from build123d import *

# Parameters (mm, degrees)
EXTRUDE_THIN1_DEPTH = 101.6
CUT_EXTRUDE1_DEPTH  = 49.784
LPATTERN1_COUNT     = 4
LPATTERN1_PITCH     = 20.32


with BuildPart() as part:
    # Sketch1 → Extrude-Thin1 (new body)
    with BuildSketch(Plane.XY):
        with BuildLine():
            Line((0, 0), (9.525, 0))
            ThreePointArc((9.525, 0), (11.77006403, 0.92993597), (12.7, 3.175))
            Line((12.7, 3.175), (12.7, 7.984742102))
            ThreePointArc((12.7, 7.984742102), (13.62993597, 10.229806132), (15.875, 11.159742102))
            Line((15.875, 11.159742102), (85.725, 11.159742102))
            ThreePointArc((85.725, 11.159742102), (87.97006403, 10.229806132), (88.9, 7.984742102))
            Line((88.9, 7.984742102), (88.9, 3.175))
            ThreePointArc((88.9, 3.175), (89.82993597, 0.92993597), (92.075, 0))
            Line((92.075, 0), (101.6, 0))
            Line((101.6, 0), (101.6, -2.032))
            Line((101.6, -2.032), (92.075, -2.032))
            ThreePointArc((92.075, -2.032), (88.39309499, -0.50690501), (86.868, 3.175))
            Line((86.868, 3.175), (86.868, 7.984742102))
            ThreePointArc((86.868, 7.984742102), (86.533223051, 8.792965153), (85.725, 9.127742102))
            Line((85.725, 9.127742102), (15.875, 9.127742102))
            ThreePointArc((15.875, 9.127742102), (15.066776949, 8.792965153), (14.732, 7.984742102))
            Line((14.732, 7.984742102), (14.732, 3.175))
            ThreePointArc((14.732, 3.175), (13.20690501, -0.50690501), (9.525, -2.032))
            Line((9.525, -2.032), (0, -2.032))
            Line((0, -2.032), (0, 0))
        make_face()
    extrude(amount=-EXTRUDE_THIN1_DEPTH)

    # Sketch2 → Cut-Extrude1 (cut, symmetric)
    with BuildSketch(Plane(origin=(0, 0, 0), x_dir=(1, 0, 0), z_dir=(0, 1, 0))):
        with BuildLine():
            Line((25.4, 23.495), (76.2, 23.495))
            ThreePointArc((76.2, 23.495), (79.375, 20.32), (76.2, 17.145))
            Line((76.2, 17.145), (25.4, 17.145))
            ThreePointArc((25.4, 17.145), (22.225, 20.32), (25.4, 23.495))
        make_face()
    cut_extrude1 = extrude(amount=CUT_EXTRUDE1_DEPTH, both=True, mode=Mode.SUBTRACT)

    # LPattern1: Cut-Extrude1 ×4
    with Locations(*[(0, 0, -i * LPATTERN1_PITCH) for i in range(1, LPATTERN1_COUNT)]):
        add(cut_extrude1, mode=Mode.SUBTRACT)


solid = part.part
Geometry check sheet. Reference: the model listing, model coordinates, mm. A direction names the side the tool comes from. Coordinates: 2 decimals unless noted, no trailing zeros. Order: outer loops, then holes, each group sorted by start corner. A loop starts at its lowest first (then second) coordinate and runs counter-clockwise, first axis right, second up. Notation, with made-up numbers: (36.5, 54) - (61.5, 54) arc R18 cw to (61.5, 86) - close; hole circle Ø10 at (32.25, 41). An arc over 180 degrees is marked (long way). One line per item, written item: value.
(1) Sectioned sample at D-D (z = -33). Enter the section's corners in (x, y) (3 decimals).
Data:
outline: (0, -2.032) - (9.525, -2.032) arc R5.207 ccw to (14.732, 3.175) - (14.732, 7.985) arc R1.143 cw to (15.875, 9.128) - (85.725, 9.128) arc R1.143 cw to (86.868, 7.985) - (86.868, 3.175) arc R5.207 ccw to (92.075, -2.032) - (101.6, -2.032) - (101.6, 0) - (92.075, 0) arc R3.175 cw to (88.9, 3.175) - (88.9, 7.985) arc R3.175 ccw to (85.725, 11.16) - (15.875, 11.16) arc R3.175 ccw to (12.7, 7.985) - (12.7, 3.175) arc R3.175 cw to (9.525, 0) - (0, 0) - close
(2) Release check for a two-part mould opening along Z. For faces 6 (the face through (79.374, 10.158, -20.39)), 7 (the face through (5, 0, -50)), 8 (the face through (51, 9.5, 0)), 9 (the face through (79.374, 10.158, -81.35)) record: +Z half, -Z half, draft (parallel to the pull), parting line (faces both ways), or undercut.
Data:
face 6: undercut
face 7: draft
face 8: +Z half
face 9: undercut
(3) Thickness scan on probe 1 along X at (y, z) = (5.75, -88.5); probe 2 along Y at (x, z) = (43, -29); probe 3 along X at (y, z) = (0.5, -79). Record the ranges inside material, lowest first. Write a range as from..to.
Data:
probe 1: x = 12.7..14.73, 86.87..88.9
probe 2: y = 9.13..11.16
probe 3: x = 11.24..13.99, 87.61..90.36
(4) Sectioned sample at C-C (z = -60.96). Enter the section's corners in (x, y) (3 decimals).
Data:
outline: (0, -2.032) - (9.525, -2.032) arc R5.207 ccw to (14.732, 3.175) - (14.732, 7.985) arc R1.143 cw to (15.875, 9.128) - (22.225, 9.128) - (22.225, 11.16) - (15.875, 11.16) arc R3.175 ccw to (12.7, 7.985) - (12.7, 3.175) arc R3.175 cw to (9.525, 0) - (0, 0) - close; (79.375, 9.128) - (85.725, 9.128) arc R1.143 cw to (86.868, 7.985) - (86.868, 3.175) arc R5.207 ccw to (92.075, -2.032) - (101.6, -2.032) - (101.6, 0) - (92.075, 0) arc R3.175 cw to (88.9, 3.175) - (88.9, 7.985) arc R3.175 ccw to (85.725, 11.16) - (79.375, 11.16) - close
(5) Sectioned sample at A-A (x = 47). Enter the section's corners in (y, z) (3 decimals).
Data:
outline: (9.128, -101.6) - (11.16, -101.6) - (11.16, -84.455) - (9.128, -84.455) - close; (9.128, -78.105) - (11.16, -78.105) - (11.16, -64.135) - (9.128, -64.135) - close; (9.128, -57.785) - (11.16, -57.785) - (11.16, -43.815) - (9.128, -43.815) - close; (9.128, -37.465) - (11.16, -37.465) - (11.16, -23.495) - (9.128, -23.495) - close; (9.128, -17.145) - (11.16, -17.145) - (11.16, 0) - (9.128, 0) - close
(6) Depth check by flat-ended pin: pin 1 Ø10.5 at (x, z) = (4, -49.5) entering from +Y; pin 2 Ø1.5 at (x, z) = (50, -59.5) entering from +Y; pin 3 Ø21 at (x, z) = (61, -44) entering from -Y; pin 4 Ø3 at (y, z) = (8.5, -15) entering from +X. Enter the tip coordinate at first touch or a pass-through.
Data:
pin 1: stops at y = 0
pin 2: passes through
pin 3: stops at y = 9.13
pin 4: stops at x = 88.9
(7) Access from +Z, -Z, +X, -X, +Y, -Y to the whole of each face (thin tool, end or side, straight path). Record for faces 1 (the face through (22.226, 10.158, -60.89)), 2 (the face through (12.7, 6, -50)), 3 (the face through (5, -2.032, -50)), 4 (the face through (86.868, 6, -50)), 5 (the face through (97, 0, -50)).
Data:
face 1: +Y, -Y
face 2: +Z, -Z, -X, +Y
face 3: +Z, -Z, +X, -X, -Y
face 4: +Z, -Z, -Y
face 5: +Z, -Z, +X, +Y
(8) Sectioned sample at B-B (y = 5.5). Enter the section's corners in (x, z).
Data:
outline: (12.7, -101.6) - (14.73, -101.6) - (14.73, 0) - (12.7, 0) - close; (86.87, -101.6) - (88.9, -101.6) - (88.9, 0) - (86.87, 0) - close
